from build123d import *

# Parameters (mm, degrees)
F0_R     = 2.1
F0_R_2   = 36.5
F1_DEPTH = 8
F2_SIZE  = 0.5


with BuildPart() as f1:
    # F0 (on Top) → F1 (new body)
    with BuildSketch(Plane.XY):
        Polygon((-37, 45), (-132, 45), (-132, -45), (-37, -45), (-12, -45), (-12, 0), (-12, 45), align=None)
        with Locations((-118.8, -34.8)):
            Circle(F0_R, mode=Mode.SUBTRACT)
        with Locations((-49.2, -34.8)):
            Circle(F0_R, mode=Mode.SUBTRACT)
        with Locations((-84, 0)):
            Circle(F0_R_2, mode=Mode.SUBTRACT)
        with Locations((-118.8, 34.8)):
            Circle(F0_R, mode=Mode.SUBTRACT)
        with BuildLine():
            ThreePointArc((-29, 30), (-24, 35), (-19, 30))
            Line((-19, 30), (-19, -30))
            ThreePointArc((-19, -30), (-24, -35), (-29, -30))
            Line((-29, -30), (-29, 30))
        make_face(mode=Mode.SUBTRACT)
        with Locations((-49.2, 34.8)):
            Circle(F0_R, mode=Mode.SUBTRACT)
    extrude(amount=F1_DEPTH)

    # F2
    f2_edges = [f1.edges().sort_by_distance(p)[0] for p in [
        (-47.5, 0, 4),
        (-120.5, 0, 0),
        (-120.5, 0, 8),
        (-116.7, -34.8, 4),
        (-120.9, -34.8, 0),
        (-120.9, -34.8, 8),
        (-116.7, 34.8, 4),
        (-120.9, 34.8, 0),
        (-120.9, 34.8, 8),
        (-47.1, 34.8, 4),
        (-51.3, 34.8, 0),
        (-51.3, 34.8, 8),
        (-47.1, -34.8, 4),
        (-51.3, -34.8, 0),
        (-51.3, -34.8, 8),
    ]]
    chamfer(f2_edges, length=F2_SIZE)


solid = f1.part
The model under review builds one solid part; all positions refer to its coordinate system, in mm. A direction names the side the tool comes from. Round coordinates to 2 decimals unless told otherwise and drop trailing zeros. Loops run counter-clockwise (first coordinate to the right, second up) from the corner with the lowest first, then second, coordinate; pieces in that order, holes last. Notation, with made-up numbers: (62, 13) -> (100, 13) arc R24 cw to (100, 24) -> close; hole circle Ø1 at (81.25, 56.5). An arc over 180 degrees is marked (long way). One line per question, with ' | ' between items. Start each with the question number.
Item 1: Add section A-A, the plane z = 6. Write out the cut boundary in (x, y), then the cut area to 3 significant figures.
Item 2: Draft analysis for pull direction Y (two halves, no side actions). For faces 3 (the face through (-24, 35, 4)), 4 (the face through (-71, 45, 4)), 5 (the face through (-49.473, 36.882, 3.951)), 6 (the face through (-132, 1, 4)), state which applies: +Y half, -Y half, draft (parallel to the pull), parting line (faces both ways), or undercut.
Item 3: Machinability: for faces 1 (the face through (-19, 0, 4)), 2 (the face through (-46, 1, 8)), which of the approach directions +Z, -Z, +X, -X, +Y, -Y give a long, thin tool a straight path to every point of the face, cutting with its end or side? Answer none if there is none.
Item 4: For pin 1 (3.5 mm diameter, centred on x = -118.8, y = -34.8, fed in from -Z); pin 2 (5 mm diameter, centred on x = -118.8, y = 34.8, fed in from -Z), all flat-tipped, find the tip position at first contact; note any pin that passes through.
Item 5: Wall thickness on line 1 along Y through (x, z) = (-24, 4.5); line 2 along Y through (x, z) = (-84, 3.75); line 3 along X through (y, z) = (-28.5, 3.75): over which ranges is each line inside the solid? List them lowest first. Write a range as [from, to].
Item 6: Add section B-B, the plane x = -118.8. Count the separate pieces of the cut face and the enclosed holes in it, then the cut area to 3 significant figures.
Return value:
1) outline: (-132, -45) -> (-12, -45) -> (-12, 45) -> (-132, 45) -> close; hole circle Ø4.2 at (-118.8, -34.8); hole circle Ø4.2 at (-118.8, 34.8); hole circle Ø73 at (-84, 0); hole circle Ø4.2 at (-49.2, -34.8); hole circle Ø4.2 at (-49.2, 34.8); hole (-29, -30) arc R5 ccw to (-19, -30) -> (-19, 30) arc R5 ccw to (-29, 30) -> close | area: 5,880 mm2
2) face 3: undercut | face 4: +Y half | face 5: undercut | face 6: draft
3) face 1: +Z, -Z | face 2: +Z, +X, -X, +Y, -Y
4) pin 1: passes through | pin 2: stops at z = 0.1
5) line 1: y = [-45, -35], [35, 45] | line 2: y = [-45, -36.5], [36.5, 45] | line 3: x = [-132, -106.8], [-61.2, -29], [-19, -12]
6) separate pieces: 4 | enclosed holes: 0 | area: 474 mm2
